Work out the finished part from the listing and answer in its coordinate system (mm). Face numbers are marked on the shaded views. A direction names the side the tool comes from. Give positions to 0.01 mm unless a question says otherwise; leave off trailing zeros. Write each loop counter-clockwise with the first axis right and the second up, starting at its lowest first coordinate (ties: lowest second). Pieces come first, ordered by that corner, then holes.
1) A tool of negligible diameter and unlimited length cuts with its end or side. For the marked faces 5 and 6, from which of +Z, -Z, +X, -X, +Y, -Y can it reach the whole face along a straight path? Write none if from no direction.
2) Find section C-C (y = -2.75). Determine the outline of the cut face in (x, z), plus the area to 3 significant figures.
3) Determine the mould class of the marked faces 1, 2, 3 and 4 for opening direction Y: pulls with the +Y half, pulls with the -Y half, needs draft (parallel to the pull), parting line crosses it, or undercut.
4) Given pin 1 Ø4 at (x, z) = (-1.5, -2.5) entering from +Y; pin 2 Ø4 at (x, z) = (1, -2.5) entering from -Y; pin 3 Ø2 at (x, y) = (-1.5, -4.5) entering from -Z, each flat-ended and moving along its own axis, determine where each tip first touches the part or whether it passes through.
5) Straight lines are drawn through the part: probe 1 along Z at (x, y) = (2.25, 3); probe 2 along Y at (x, z) = (-0.25, -2.25); probe 3 along Y at (x, z) = (-0.75, -0.5). For each, find the intervals that lie inside material, in ascending order.
6) Find section A-A (z = -3.5). Determine the outline of the cut face in (x, y).
7) Find section D-D (z = 0.5). Determine the outline of the cut face in (x, y).
8) Find section B-B (x = 1.25). Determine the outline of the cut face in (y, z), plus the area to 3 significant figures.
```python
from build123d import *
from build123d import SkipClean  # not in build123d's __all__

# Parameters (mm, degrees)
F1_DEPTH = 2
F2_DEPTH = 6


with BuildPart() as f1:
    # F0 (on Top) → F1 (new body)
    with BuildSketch(Plane.XY):
        with BuildLine():
            Line((-2.522197513, 2.4266272284), (-3.1941037004, -1.430979228))
            ThreePointArc((-3.1941037004, -1.430979228), (0, -3.5), (3.1941037004, -1.430979228))
            Line((3.1941037004, -1.430979228), (2.522197513, 2.4266272284))
            ThreePointArc((2.522197513, 2.4266272284), (0, 3.5), (-2.522197513, 2.4266272284))
        make_face()
        with BuildLine():
            ThreePointArc((2, 1.5), (2.3717082451, 0.790569415), (2.5, 0))
            ThreePointArc((2.5, 0), (2.3717082451, -0.790569415), (2, -1.5))
            ThreePointArc((2, -1.5), (0, -2.5), (-2, -1.5))
            ThreePointArc((-2, -1.5), (-2.5, 0), (-2, 1.5))
            ThreePointArc((-2, 1.5), (0, 2.5), (2, 1.5))
        make_face(mode=Mode.SUBTRACT)
        with BuildLine():
            Line((0, 16.9072877616), (-2.522197513, 2.4266272284))
            ThreePointArc((-2.522197513, 2.4266272284), (0, 3.5), (2.522197513, 2.4266272284))
            Line((2.522197513, 2.4266272284), (0, 16.9072877616))
        make_face()
        with BuildLine():
            Line((-3.1941037004, -1.430979228), (-3.7119607441, -4.4041452929))
            ThreePointArc((-3.7119607441, -4.4041452929), (0, -5.7597871772), (3.7119607441, -4.4041452929))
            Line((3.7119607441, -4.4041452929), (3.1941037004, -1.430979228))
            ThreePointArc((3.1941037004, -1.430979228), (0, -3.5), (-3.1941037004, -1.430979228))
        make_face()
        with BuildLine():
            ThreePointArc((2, -1.5), (2.3717082451, -0.790569415), (2.5, 0))
            ThreePointArc((2.5, 0), (2.3717082451, 0.790569415), (2, 1.5))
            Line((2, 1.5), (-2, 1.5))
            ThreePointArc((-2, 1.5), (-2.5, 0), (-2, -1.5))
            Line((-2, -1.5), (2, -1.5))
        make_face()
        with BuildLine():
            Line((-2, 1.5), (2, 1.5))
            ThreePointArc((2, 1.5), (0, 2.5), (-2, 1.5))
        make_face()
        with BuildLine():
            ThreePointArc((-2, -1.5), (0, -2.5), (2, -1.5))
            Line((2, -1.5), (-2, -1.5))
        make_face()
        with BuildLine():
            Line((2.522197513, 2.4266272284), (3.1941037004, -1.430979228))
            ThreePointArc((3.1941037004, -1.430979228), (3.4226716868, -0.7316546482), (3.5, 0))
            ThreePointArc((3.5, 0), (3.2463588292, 1.3081109862), (2.522197513, 2.4266272284))
        make_face()
        with BuildLine():
            ThreePointArc((-2.522197513, 2.4266272284), (-3.4480874095, 0.6005774025), (-3.1941037004, -1.430979228))
            Line((-3.1941037004, -1.430979228), (-2.522197513, 2.4266272284))
        make_face()
    extrude(amount=F1_DEPTH)

    # F0 (on Top) → F2 (join)
    with BuildSketch(Plane.XY):
        with BuildLine():
            ThreePointArc((-2.522197513, 2.4266272284), (-3.4480874095, 0.6005774025), (-3.1941037004, -1.430979228))
            Line((-3.1941037004, -1.430979228), (-2.522197513, 2.4266272284))
        make_face()
        with BuildLine():
            Line((2.522197513, 2.4266272284), (3.1941037004, -1.430979228))
            ThreePointArc((3.1941037004, -1.430979228), (3.4226716868, -0.7316546482), (3.5, 0))
            ThreePointArc((3.5, 0), (3.2463588292, 1.3081109862), (2.522197513, 2.4266272284))
        make_face()
        with BuildLine():
            Line((-2.522197513, 2.4266272284), (-3.1941037004, -1.430979228))
            ThreePointArc((-3.1941037004, -1.430979228), (0, -3.5), (3.1941037004, -1.430979228))
            Line((3.1941037004, -1.430979228), (2.522197513, 2.4266272284))
            ThreePointArc((2.522197513, 2.4266272284), (0, 3.5), (-2.522197513, 2.4266272284))
        make_face()
        with BuildLine():
            ThreePointArc((2, 1.5), (2.3717082451, 0.790569415), (2.5, 0))
            ThreePointArc((2.5, 0), (2.3717082451, -0.790569415), (2, -1.5))
            ThreePointArc((2, -1.5), (0, -2.5), (-2, -1.5))
            ThreePointArc((-2, -1.5), (-2.5, 0), (-2, 1.5))
            ThreePointArc((-2, 1.5), (0, 2.5), (2, 1.5))
        make_face(mode=Mode.SUBTRACT)
        with BuildLine():
            Line((-2, 1.5), (2, 1.5))
            ThreePointArc((2, 1.5), (0, 2.5), (-2, 1.5))
        make_face()
        with BuildLine():
            ThreePointArc((-2, -1.5), (0, -2.5), (2, -1.5))
            Line((2, -1.5), (-2, -1.5))
        make_face()
    with SkipClean():  # cleaning this boolean's faces spoils the solid; the shape is the same uncleaned
        extrude(amount=-F2_DEPTH)


solid = f1.part
```
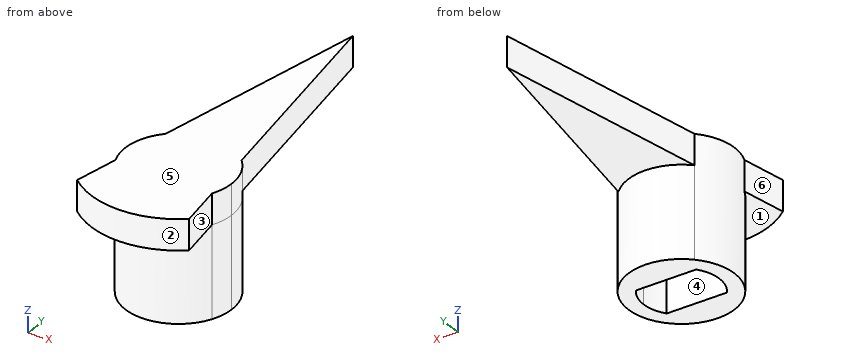
Results:
1. face 5: +Z, +X, -X, +Y, -Y
1. face 6: +Z, -Z, -X
2. outline: (-3.42, 0) - (-2.17, 0) - (-2.17, -6) - (2.17, -6) - (2.17, 0) - (3.42, 0) - (3.42, 2) - (-3.42, 2) - close
2. area: 39.7 mm2
3. face 1: needs draft
3. face 2: pulls with the -Y half
3. face 3: undercut
3. face 4: undercut
4. pin 1: stops at y = 3.5
4. pin 2: stops at y = -3.5
4. pin 3: stops at z = 0
5. probe 1: z = 0 to 2
5. probe 2: y = -3.49 to -1.5, 1.5 to 3.49
5. probe 3: y = -3.42 to -1.5, 1.5 to 3.42
6. outline: circle Ø7 at (0, 0); hole (-2, -1.5) - (2, -1.5) arc R2.5 ccw to (2, 1.5) - (-2, 1.5) arc R2.5 ccw to start
7. outline: (-3.71, -4.4) arc R5.76 ccw to (3.71, -4.4) - (3.19, -1.43) arc R3.5 ccw to (2.52, 2.43) - (0, 16.91) - (-2.52, 2.43) arc R3.5 ccw to (-3.19, -1.43) - close
8. outline: (-5.62, 0) - (-3.27, 0) - (-3.27, -6) - (-1.5, -6) - (-1.5, 0) - (1.5, 0) - (1.5, -6) - (3.27, -6) - (3.27, 0) - (9.73, 0) - (9.73, 2) - (-5.62, 2) - close
8. area: 51.9 mm2
